from build123d import *

# Parameters (mm, degrees)
CORTAR_EXTRUIR1_DEPTH = 7
REDONDEO1_R           = 1


with BuildPart() as part:
    # Croquis1 → Revolución2 (revolve)
    with BuildSketch(Plane.XY):
        Polygon((-5, 31.216383588), (-5, 11.216383588), (-8, 11.216383588), (-8, 0), (0, 0), (0, 31.772433039), (-4.288289157, 31.772433039), align=None)
    revolve(axis=Axis((0, 0, 0), (0, 1, 0)))

    # Croquis2 → Cortar-Extruir1 (cut)
    with BuildSketch(Plane.XZ):
        Polygon((0, 5.196152423), (-4.5, 2.598076211), (-4.5, -2.598076211), (0, -5.196152423), (4.5, -2.598076211), (4.5, 2.598076211), align=None)
    extrude(amount=-CORTAR_EXTRUIR1_DEPTH, mode=Mode.SUBTRACT)

    # Redondeo1
    redondeo1_edges = [part.edges().sort_by_distance(p)[0] for p in [
        (8, 11.216383588, 0),
        (8, 0, 0),
    ]]
    fillet(redondeo1_edges, radius=REDONDEO1_R)


solid = part.part
The listing builds one solid part. Answer for the finished solid, in the listing's coordinates (mm). A direction names the side the tool comes from. Give positions to 0.01 mm unless a question says otherwise; leave off trailing zeros. Loops run counter-clockwise (first coordinate to the right, second up) from the corner with the lowest first, then second, coordinate; pieces in that order, holes last. Notation, with made-up numbers: M 23.25,22 L 82.25,22 A16 ccw 82.25,53 Z; hole C 16,-7.5 d10. An arc over 180 degrees is marked long. Answer as CSV lines item,"result".
Item 1: Which of the six approach directions +Z, -Z, +X, -X, +Y, -Y give full straight-line access (tool end or side, diameter ignored) to faces 4 (the cylindrical face through (1.73, 5.54, -7.81)), 5 (the flat face through (-2, 11.216, 5)), 6 (the flat face through (-4.5, 3, 0))?
Values follow:
face 4,"+Y, -Y"
face 5,"+Y"
face 6,"-Y"
Item 2: The part is cut by section A-A (z = 0). Give the vertices of the cut face in (x, y).
Values follow:
outline,"M -8,1 A1 ccw -7,0 L -4.5,0 L -4.5,7 L 4.5,7 L 4.5,0 L 7,0 A1 ccw 8,1 L 8,10.22 A1 ccw 7,11.22 L 5,11.22 L 5,31.22 L 4.29,31.77 L -4.29,31.77 L -5,31.22 L -5,11.22 L -7,11.22 A1 ccw -8,10.22 Z"
Item 3: Given pin 1 Ø6 at (x, y) = (-2.5, 28) entering from +Z; pin 2 Ø3 at (x, z) = (-0.5, 6) entering from +Y; pin 3 Ø3 at (x, y) = (-5.5, 14.5) entering from +Z, each flat-ended and moving along its own axis, determine where each tip first touches the part or whether it passes through.
Values follow:
pin 1,"stops at z = 5"
pin 2,"stops at y = 31.59"
pin 3,"stops at z = 3"
Item 4: The part is cut by section B-B (y = 14.5). Give the vertices of the cut face in (x, z).
Values follow:
outline,"C 0,0 d10"
Item 5: Straight lines are drawn through the part: line 1 along Y through (x, z) = (0.75, -2.75); line 2 along Y through (x, z) = (-4, -3.25); line 3 along Z through (x, y) = (-2.25, 1.5). For each, find the intervals that lie inside material, in ascending order. Write a range as [from, to].
Values follow:
line 1,"y = [7, 31.77]"
line 2,"y = [0, 11.22]"
line 3,"z = [-7.68, -3.9], [3.9, 7.68]"
Item 6: The mould has two halves that part along X. Classify faces 1 (the flat face through (0, 7, 0)), 2 (the flat face through (0, 31.772, 0)), 3 (the cylindrical face through (1.08, 21.08, -4.88)): released by +X, released by -X, zero draft, split by the parting line, or undercut.
Values follow:
face 1,"undercut"
face 2,"zero draft"
face 3,"split by the parting line"
